Design review of the part built by this model. Coordinates are the model's own, in mm. A direction names the side the tool comes from. Coordinates: 2 decimals unless noted, no trailing zeros. Write each loop counter-clockwise with the first axis right and the second up, starting at its lowest first coordinate (ties: lowest second). Pieces come first, ordered by that corner, then holes.
Q1. The part is to be moulded in two halves that separate along Y. For faces 1 (the face through (-25.4, 61.4, 23.3)), 2 (the face through (-0.36, 72.22, 13.65)), 3 (the face through (-38, 101.6, 1)), say which applies: +Y half, -Y half, draft (parallel to the pull), parting line (faces both ways), or undercut.
Q2. Clearance check with a flat-ended pin moving along its axis: pin 1 Ø2 at (x, z) = (28, 39.5) entering from -Y. State where the tip first meets the part, or that it passes through.
Q3. Add section B-B, the plane z = 11. Give the boundary of the cut face in (x, y), plus the area to 3 significant figures.
Q4. Add section C-C, the plane z = -31.5. Give the boundary of the cut face in (x, y), plus the area to 3 significant figures.
Q5. To check wall thickness, follow probe 1 along Z at (x, y) = (1, 50); probe 2 along Y at (x, z) = (-13, 0); probe 3 along X at (y, z) = (25.5, 37). State the ranges of each line that lie inside material, in increasing order.
Q6. Machinability: for faces 4 (the face through (25.4, 61.4, 23.3)), 5 (the face through (-1, 251, -50.8)), which of the approach directions +Z, -Z, +X, -X, +Y, -Y give a long, thin tool a straight path to every point of the face, cutting with its end or side? Answer none if there is none.
from build123d import *

# Parameters (mm, degrees)
SKETCH1_W           = 101.6
SKETCH1_H           = 101.6
BOSS_EXTRUDE1_DEPTH = 457.2
SKETCH2_W           = 25.4
SKETCH2_H           = 101.6
CUT_EXTRUDE1_DEPTH  = 472.099819571
FILLET1_R           = 50.8
SKETCH3_R           = 25.4
CUT_EXTRUDE2_DEPTH  = 467.282017667


with BuildPart() as part:
    # Sketch1 → Boss-Extrude1 (new body)
    with BuildSketch(Plane(origin=(0, 0, 0), x_dir=(1, 0, 0), z_dir=(0, 1, 0))):
        Rectangle(SKETCH1_W, SKETCH1_H)
    extrude(amount=BOSS_EXTRUDE1_DEPTH)

    # Sketch2 → Cut-Extrude1 (cut, through all)
    with BuildSketch(Plane.XY.offset(50.8)):
        with Locations((-38.1, 50.8)):
            Rectangle(SKETCH2_W, SKETCH2_H)
        with Locations((38.1, 50.8)):
            Rectangle(SKETCH2_W, SKETCH2_H)
    extrude(amount=-CUT_EXTRUDE1_DEPTH, mode=Mode.SUBTRACT)

    # Fillet1
    fillet1_edges = [part.edges().sort_by_distance(p)[0] for p in [
        (0, 0, -50.8),
        (0, 0, 50.8),
    ]]
    fillet(fillet1_edges, radius=FILLET1_R - 0.0001)  # a hair under: the kernel refuses the full size

    # Sketch3 → Cut-Extrude2 (cut, through all)
    with BuildSketch(Plane.ZY.offset(25.4)):
        with Locations((0, 50.8)):
            Circle(SKETCH3_R)
    extrude(amount=-CUT_EXTRUDE2_DEPTH, mode=Mode.SUBTRACT)


solid = part.part
Here are the results:
1. face 1: draft
1. face 2: undercut
1. face 3: -Y half
2. pin 1: stops at y = 101.6
3. outline: (-50.8, 101.6) - (-25.4, 101.6) - (-25.4, 73.69) - (25.4, 73.69) - (25.4, 101.6) - (50.8, 101.6) - (50.8, 457.2) - (-50.8, 457.2) - close; (-25.4, 1.21) - (25.4, 1.21) - (25.4, 27.91) - (-25.4, 27.91) - close
3. area: 38,900 mm2
4. outline: (-50.8, 101.6) - (-25.4, 101.6) - (-25.4, 10.95) - (25.4, 10.95) - (25.4, 101.6) - (50.8, 101.6) - (50.8, 457.2) - (-50.8, 457.2) - close
4. area: 40,700 mm2
5. probe 1: z = -50.79 to -25.39, 25.39 to 50.79
5. probe 2: y = 0 to 25.4, 76.2 to 457.2
5. probe 3: x = -25.4 to 25.4
6. face 4: +Z, -Z, +X, -Y
6. face 5: -Z, +X, -X, +Y, -Y
